The listing builds one solid part. Answer for the finished solid, in the listing's coordinates (mm). A direction names the side the tool comes from. Coordinates: 2 decimals unless noted, no trailing zeros. Loops run counter-clockwise (first coordinate to the right, second up) from the corner with the lowest first, then second, coordinate; pieces in that order, holes last. Notation, with made-up numbers: (83.25, 78) - (87.25, 78) arc R28 ccw to (87.25, 110) - close; hole circle Ø7 at (64, -26.5). An arc over 180 degrees is marked (long way). Put each result on its own line as item: value.
Autodesk Inventor part; units mm, degrees
ref_plane "Start plane" through (0, 0, 50) normal (0, 0, 1) x (1, 0, 0)
ref_plane "End plane" through (0, 0, 360) normal (0, 0, 1) x (1, 0, 0)
ref_plane "Work Plane4" through (-9.2, 565, 50) normal (0, 0, -1) x (-1, 0, 0)
ref_plane "Start plane" through (0, 0, 50) normal (0, 0, 1) x (1, 0, 0)
ref_plane "End plane" through (0, 0, 360) normal (0, 0, 1) x (1, 0, 0)
sketch "Sketch" plane through (0, 0, 0) normal (0, 0, 1) x (1, 0, 0)
  line L0 (-20, -13.4) -> (-20, 13.4)
  line L1 (-13.4, 20) -> (13.4, 20)
  line L2 (20, 13.4) -> (20, -13.4)
  line L3 (13.4, -20) -> (-13.4, -20)
  arc A0 (-20, -13.4) -> (-13.4, -20) centre (-13.4, -13.4) ccw
  arc A1 (-13.4, 20) -> (-20, 13.4) centre (-13.4, 13.4) ccw
  arc A2 (20, 13.4) -> (13.4, 20) centre (13.4, 13.4) ccw
  arc A3 (13.4, -20) -> (20, -13.4) centre (13.4, -13.4) ccw
  arc A4 (-13.4, 17) -> (-17, 13.4) centre (-13.4, 13.4) ccw
  line L4 (-13.4, 17) -> (13.4, 17)
  arc A5 (17, 13.4) -> (13.4, 17) centre (13.4, 13.4) ccw
  line L5 (17, 13.4) -> (17, -13.4)
  arc A6 (13.4, -17) -> (17, -13.4) centre (13.4, -13.4) ccw
  line L6 (13.4, -17) -> (-13.4, -17)
  arc A7 (-17, -13.4) -> (-13.4, -17) centre (-13.4, -13.4) ccw
  line L7 (-17, -13.4) -> (-17, 13.4)
  line L8 (0, 22.0873) -> (0, -22.0873) construction
  line L9 (-22.0873, 0) -> (22.0873, 0) construction
  dimension "d7" = 6.6
  dimension "d10" = 40
  dimension "d11" = 40
  dimension "d12" = 3
  dimension "d15" = 20
  dimension "d16" = 20
extrude "Body" add sketch "Sketch" along normal up to surface (310 mm away) from surface at 50
sketch "Sketch3" plane through (0, 0, 0) normal (0, 0, 1) x (1, 0, 0)
  line L0 (0, 0) -> (10, 0)
ref_plane "Work Plane3" through (0, 0, 0) normal (0, -1, 0) x (1, 0, 0)
sketch "Sketch4" plane through (0, 0, 0) normal (0, -1, 0) x (1, 0, 0)
  line L0 (-2, 50) -> (12, 50)
  line L1 (-2, 360) -> (12, 360)
  dimension "d18" = 310
ref_plane "Work Plane4" through (-9.2, 565, 50) normal (0, 0, -1) x (-1, 0, 0)
split "Split1" plane through (-9.2, 565, 50) removes the side toward (0, 0, -1)
ref_plane "Work Plane5" through (636, -8.4, 360) normal (0, 0, 1) x (1, 0, 0)
split "Split2" plane through (636, -8.4, 360) removes the side toward (0, 0, 1)
equation "\"d7\" = G_IR"
equation "\"d10\" = G_H"
equation "\"d11\" = G_W"
equation "\"d12\" = G_T"
equation "\"d15\" = 0.5 * d10"
equation "\"d16\" = 0.5 * d11"
equation "\"d3\" = G_L"
equation "\"G_W\" = 40"
equation "\"G_H\" = 40"
equation "\"G_T\" = 3"
equation "\"G_IR\" = 6.6"
equation "\"G_L\" = d18"
properties part number "DIN EN 10305-5 - 40 x 40 x 3  - 310" material "Steel, Mild"
1) Straight lines are drawn through the part: L1, parallel to X at y = -4.5, z = 233.5; L2, parallel to Y at x = 16, z = 162.5. For each, find the intervals that lie inside material, in ascending order. Write a range as [from, to].
Found:
L1: x = [-20, -17], [17, 20]
L2: y = [-19.47, -15.89], [15.89, 19.47]
2) For a pull along X with two mould halves and no side action, classify faces 3 (the face through (0, 17, 203)), 4 (the face through (18.118, -18.015, 202.83)), 5 (the face through (-20, 0, 203)), 6 (the face through (0, 20, 203)) as pulls with the +X half, pulls with the -X half, needs draft (parallel to the pull), parting line crosses it, or undercut.
Found:
face 3: undercut
face 4: pulls with the +X half
face 5: pulls with the -X half
face 6: needs draft
3) The part is cut by section A-A (x = -5). Give the vertices of the cut face in (y, z).
Found:
outline: (-20, 50) - (-17, 50) - (-17, 360) - (-20, 360) - close; (17, 50) - (20, 50) - (20, 360) - (17, 360) - close
4) This flat-tipped pin is pushed along its axis until it touches: pin 1 (2 mm diameter, centred on x = -13, y = -14.5, fed in from -Z). Where does it stop, or does it pass through?
Found:
pin 1: passes through
5) The part is cut by section B-B (z = 102). Give the vertices of the cut face in (x, y).
Found:
outline: (-20, -13.4) arc R6.6 ccw to (-13.4, -20) - (13.4, -20) arc R6.6 ccw to (20, -13.4) - (20, 13.4) arc R6.6 ccw to (13.4, 20) - (-13.4, 20) arc R6.6 ccw to (-20, 13.4) - close; hole (-17, -13.4) arc R3.6 ccw to (-13.4, -17) - (13.4, -17) arc R3.6 ccw to (17, -13.4) - (17, 13.4) arc R3.6 ccw to (13.4, 17) - (-13.4, 17) arc R3.6 ccw to (-17, 13.4) - close
6) For faces 1 (the face through (17, 0, 203)), 2 (the face through (18.015, 18.118, 202.83)), determine the directions among +Z, -Z, +X, -X, +Y, -Y from which every point of the face is accessible in a straight line to the end or side of a thin tool.
Found:
face 1: +Z, -Z
face 2: +Z, -Z, +X, +Y
